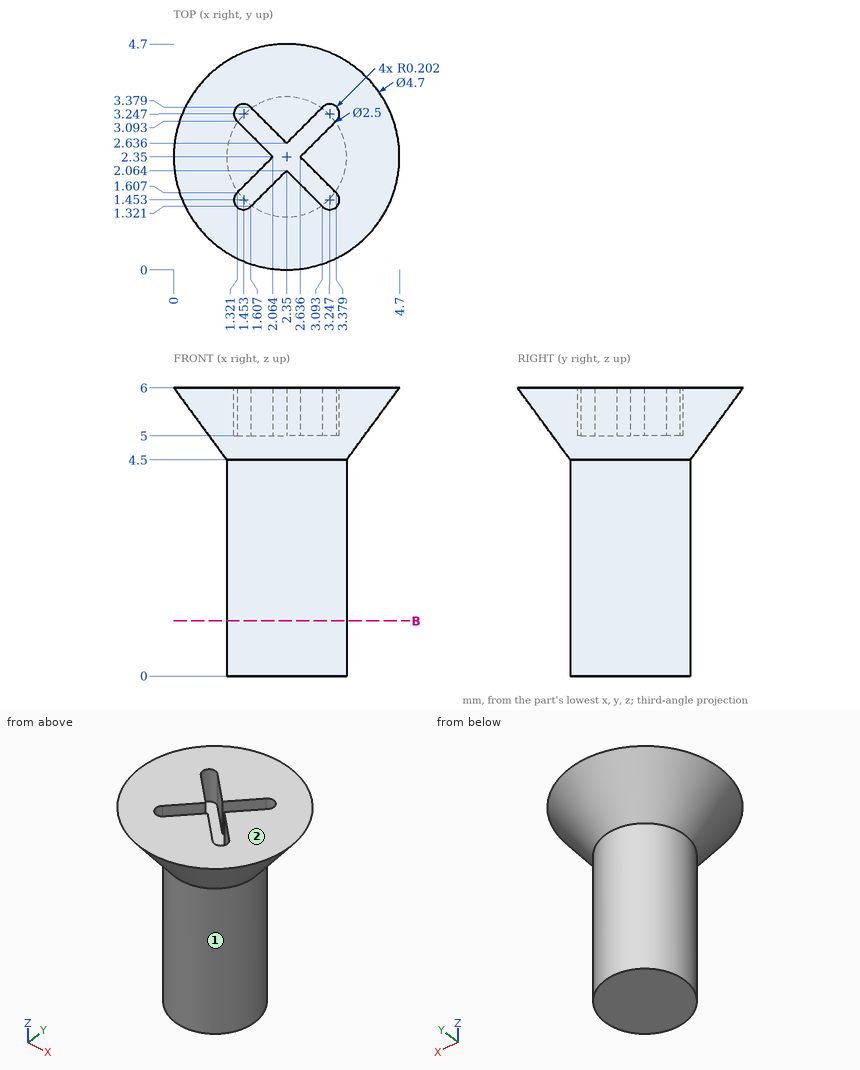
The figure shows three views and two pictorial views of one solid part (mm, origin at its lowest corner). Answer the questions. A direction names the side the tool comes from. Give positions to 0.01 mm unless a question says otherwise; leave off trailing zeros. Write each loop counter-clockwise with the first axis right and the second up, starting at its lowest first coordinate (ties: lowest second). Pieces come first, ordered by that corner, then holes. Notation, with made-up numbers: (-35, 58) -> (-8, 58) arc R11 cw to (-8, 65) -> close; hole circle Ø7 at (52.5, -10.5). An arc over 180 degrees is marked (long way). Answer as a JSON object with one key per item and string values.
1) Straight lines are drawn through the part: probe 1 along Y at (x, z) = (2.4, 2.05); probe 2 along X at (y, z) = (2.9, 5.5) (1 decimal); probe 3 along Z at (x, y) = (3.2, 1.4) (1 decimal). For each, find the intervals that lie inside material, in ascending order. Write a range as from..to.
Findings below:
{"probe 1": "y = 1.1..3.6", "probe 2": "x = 0.4..1.5, 2.1..2.6, 3.2..4.3", "probe 3": "z = 4.5..5"}
2) Section B-B on z = 1.15 is taken. Write down the section's boundary in (x, y).
Findings below:
{"outline": "circle Ø2.5 at (2.35, 2.35)"}
3) A tool of negligible diameter and unlimited length cuts with its end or side. For the marked faces 1 and 2, from which of +Z, -Z, +X, -X, +Y, -Y can it reach the whole face along a straight path? Write none if from no direction.
Findings below:
{"face 1": "-Z", "face 2": "+Z, +X, -X, +Y, -Y"}
